from build123d import *

# Parameters (mm, degrees)
SKETCH_1_R      = 2
SKETCH_1_W      = 8
SKETCH_1_H      = 8
EXTRUDE_1_DEPTH = 4


with BuildPart() as part:
    # 草图1 → 凸台-拉伸1 (new, symmetric)
    with BuildSketch(Plane(origin=(0, 0, 0), x_dir=(0, 0, -1), z_dir=(1, 0, 0))):
        with BuildLine():
            Line((-28.857142857, 5.938459912), (-1.428571429, 9.897433186))
            ThreePointArc((-1.428571429, 9.897433186), (10, 0), (-1.428571429, -9.897433186))
            Line((-1.428571429, -9.897433186), (-28.857142857, -5.938459912))
            ThreePointArc((-28.857142857, -5.938459912), (-34, 0), (-28.857142857, 5.938459912))
        make_face()
        with Locations((-28, 0)):
            Circle(SKETCH_1_R, mode=Mode.SUBTRACT)
        Rectangle(SKETCH_1_W, SKETCH_1_H, mode=Mode.SUBTRACT)
        with BuildLine():
            Line((-17.5, 2.598076211), (-16, 3.464101615))
            ThreePointArc((-16, 3.464101615), (-10, 0), (-16, -3.464101615))
            Line((-16, -3.464101615), (-17.5, -2.598076211))
            ThreePointArc((-17.5, -2.598076211), (-19, 0), (-17.5, 2.598076211))
        make_face(mode=Mode.SUBTRACT)
    extrude(amount=EXTRUDE_1_DEPTH, both=True)


solid = part.part
Check sheet for the modelled part. Datum: model origin and axes. Units: mm. A direction names the side the tool comes from. Coordinates: 2 decimals unless noted, no trailing zeros. Write each loop counter-clockwise with the first axis right and the second up, starting at its lowest first coordinate (ties: lowest second). Pieces come first, ordered by that corner, then holes.
Item 1: Cross-section at B-B on x = 1. Record the boundary of the cut face in (y, z), then the cut area to 3 significant figures.
Numbers:
outline: (-9.9, 1.43) arc R10 ccw (long way) to (9.9, 1.43) - (5.94, 28.86) arc R6 ccw to (-5.94, 28.86) - close; hole (-4, -4) - (4, -4) - (4, 4) - (-4, 4) - close; hole (-3.46, 16) arc R4 ccw (long way) to (3.46, 16) - (2.6, 17.5) arc R3 ccw to (-2.6, 17.5) - close; hole circle Ø4 at (0, 28)
area: 535 mm2
Item 2: Cross-section at D-D on z = 28. Record the boundary of the cut face in (x, y), then the cut area to 3 significant figures.
Numbers:
outline: (-4, -6.06) - (4, -6.06) - (4, -2) - (-4, -2) - close; (-4, 2) - (4, 2) - (4, 6.06) - (-4, 6.06) - close
area: 65.0 mm2
Item 3: Scan lines: probe 1 along Z at (x, y) = (0, -2.5); probe 2 along Z at (x, y) = (1.75, 3.25); probe 3 along Y at (x, z) = (3, 14). Record each from-to range of solid material in increasing order.
Numbers:
probe 1: z = -9.68 to -4, 4 to 10.88, 17.66 to 33.45
probe 2: z = -9.46 to -4, 4 to 11.67, 16.37 to 33.04
probe 3: y = -8.08 to -4, 4 to 8.08
Item 4: Depth check by flat-ended pin: pin 1 Ø4 at (x, y) = (2, -7.5) entering from -Z; pin 2 Ø1 at (x, z) = (-3, -1.5) entering from +Y; pin 3 Ø1.5 at (x, z) = (-1.5, 14.5) entering from -Y; pin 4 Ø2.5 at (y, z) = (0, 28) entering from +X. Enter the tip coordinate at first touch or a pass-through.
Numbers:
pin 1: stops at z = -8.35
pin 2: stops at y = 9.95
pin 3: stops at y = -8.12
pin 4: passes through
Item 5: Cross-section at A-A on y = 0. Record the boundary of the cut face in (x, z), then the cut area to 3 significant figures.
Numbers:
outline: (-4, -10) - (4, -10) - (4, -4) - (-4, -4) - close; (-4, 4) - (4, 4) - (4, 10) - (-4, 10) - close; (-4, 19) - (4, 19) - (4, 26) - (-4, 26) - close; (-4, 30) - (4, 30) - (4, 34) - (-4, 34) - close
area: 184 mm2
Item 6: Access from +Z, -Z, +X, -X, +Y, -Y to the whole of each face (thin tool, end or side, straight path). Record for faces 5 (the face through (4, 0, 7)), 6 (the face through (0.056, -3.037, 16.74)).
Numbers:
face 5: +Z, -Z, +X, +Y, -Y
face 6: +X, -X
Item 7: Mould release check, pull along Y, two halves, no side actions. Record for faces 1 (the face through (0.056, -7.946, 14.951)), 2 (the face through (0, 4, 0)), 3 (the face through (-4, 0, 7)), 4 (the face through (-0.056, 0.601, 26.092)): released by +Y, released by -Y, zero draft, split by the parting line, or undercut.
Numbers:
face 1: released by -Y
face 2: undercut
face 3: zero draft
face 4: undercut
Item 8: Cross-section at C-C on z = 12. Record the boundary of the cut face in (x, y).
Numbers:
outline: (-4, -8.37) - (4, -8.37) - (4, -3.46) - (-4, -3.46) - close; (-4, 3.46) - (4, 3.46) - (4, 8.37) - (-4, 8.37) - close
